from build123d import *

# Parameters (mm, degrees)
CYLINDER017_R          = 2.5
CYLINDER017_DEPTH      = 30
CYLINDER018_R          = 2.5
CYLINDER018_DEPTH      = 30
CYLINDER019_R          = 2.5
CYLINDER019_DEPTH      = 30
CYLINDER016_R          = 7.75
CYLINDER016_DEPTH      = 30
CYLINDER015_R          = 7.75
CYLINDER015_DEPTH      = 60
BOX001_W               = 20
BOX001_H               = 40
BOX001_DEPTH           = 20
CUT001_ROLL_ANGLE      = 180
CUT001_PLACEMENT_ANGLE = 90


with BuildPart() as taladros003:
    # Cylinder017 → Cylinder017 (new body)
    with BuildSketch(Plane(origin=(20, 15, 0), x_dir=(1, 0, 0), z_dir=(0, -1, 0))):
        Circle(CYLINDER017_R)
    extrude(amount=CYLINDER017_DEPTH)


with BuildPart() as taladros004:
    # Cylinder018 → Cylinder018 (new body)
    with BuildSketch(Plane(origin=(-20, 15, 0), x_dir=(1, 0, 0), z_dir=(0, -1, 0))):
        Circle(CYLINDER018_R)
    extrude(amount=CYLINDER018_DEPTH)


with BuildPart() as obj1:
    # Cylinder019 → Cylinder019 (new body)
    with BuildSketch(Plane(origin=(0, 15, 20), x_dir=(1, 0, 0), z_dir=(0, -1, 0))):
        Circle(CYLINDER019_R)
    extrude(amount=CYLINDER019_DEPTH)

    # Fusion004: union Taladros003, Taladros004
    add(taladros003.part)
    add(taladros004.part)


with BuildPart() as obj2:
    # Cylinder016 → Cylinder016 (new body)
    with BuildSketch(Plane.XY):
        Circle(CYLINDER016_R)
    extrude(amount=CYLINDER016_DEPTH)


with BuildPart() as obj3:
    # Cylinder015 → Cylinder015 (new body)
    with BuildSketch(Plane(origin=(-30, 0, 0), x_dir=(0, 0, -1), z_dir=(1, 0, 0))):
        Circle(CYLINDER015_R)
    extrude(amount=CYLINDER015_DEPTH)


with BuildPart() as obj4:
    # Box001 → Box001 (new body)
    with BuildSketch(Plane(origin=(-10, -30, -10), x_dir=(1, 0, 0), z_dir=(0, 0, 1))):
        with Locations((10, 20)):
            Rectangle(BOX001_W, BOX001_H)
    extrude(amount=BOX001_DEPTH)

    # Fusion003: union obj2, obj3
    add(obj2.part)
    add(obj3.part)

    # Cut001: cut obj1
    add(obj1.part, mode=Mode.SUBTRACT)


with BuildPart() as obj4_1:
    # Cut001 roll: moved
    add(obj4.part.rotate(Axis((0, 0, 0), (1, 0, 0)), CUT001_ROLL_ANGLE))


with BuildPart() as obj4_2:
    # Cut001 placement: moved
    add(obj4_1.part.moved(Location((11, -12, -22))).rotate(Axis((11, -12, -22), (0, 0, 1)), CUT001_PLACEMENT_ANGLE))


solid = obj4_2.part
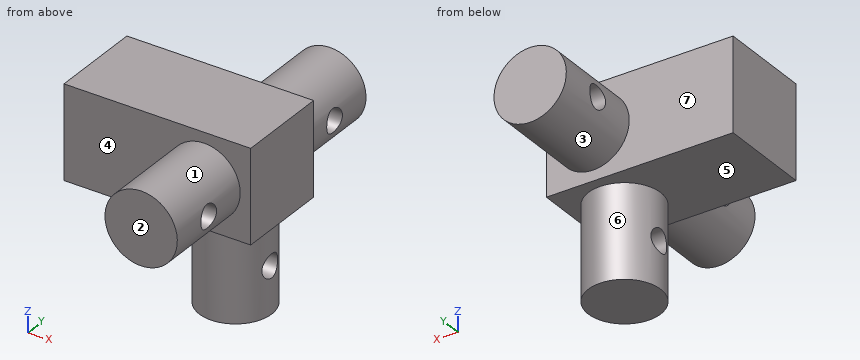
Source: CAD feature listing. Evaluate the final solid. Frame: model axes, mm. Face numbers are marked on the shaded views. A direction names the side the tool comes from. Round coordinates to 2 decimals unless told otherwise and drop trailing zeros. Order: outer loops, then holes, each group sorted by start corner. A loop starts at its lowest first (then second) coordinate and runs counter-clockwise, first axis right, second up. Notation, with made-up numbers: (-24, 11.25) - (30, 11.25) arc R19 cw to (30, 20.25) - close; hole circle Ø2 at (-0.5, -26.5). An arc over 180 degrees is marked (long way). Use a Markdown table: item, result. Add a question column.
1. Mould query, pull axis Y, two halves, no side actions, for the marked faces 4, 5, 6 and 7. Classes: +Y half, -Y half, draft (parallel to the pull), parting line (faces both ways), or undercut.
2. Section query A-A (z = -22). Return the cut outline in (x, y).
3. Section query C-C (x = 11). Return the cut outline in (y, z).
4. Section query D-D (y = -5.5). Return the cut outline in (x, z), then the cut area to 3 significant figures.
5. Set-up query: the marked faces 1, 2 and 3. Return all of +Z, -Z, +X, -X, +Y, -Y with unobstructed straight access to the full face (end or side cutting, diameter ignored); none if empty.
6. First-contact query: pin 1 (6 mm diameter, centred on y = -32, z = -22, fed in from +X); pin 2 (1.5 mm diameter, centred on x = 15, z = -36.5, fed in from +Y); pin 3 (6 mm diameter, centred on x = 0.5, z = -18.5, fed in from -Y). Flat tips, straight axial feed; report the tip coordinate or a pass-through.
7. Line query: probe 1 along Y at (x, z) = (7, -22); probe 2 along Z at (x, y) = (8.75, -12); probe 3 along Y at (x, z) = (10.5, -42). Output: solid intervals per line, ascending.
8. Section query B-B (y = -12). Return the cut outline in (x, z).
Derived:
| question | item | result |
|---|---|---|
| 1 | face 4 | -Y half |
| 1 | face 5 | draft |
| 1 | face 6 | parting line |
| 1 | face 7 | +Y half |
| 2 | outline | (-19, -22) - (3.25, -22) - (3.25, -29.5) - (18.75, -29.5) - (18.75, -22) - (21, -22) - (21, -2) - (18.75, -2) - (18.75, 5.5) - (3.25, 5.5) - (3.25, -2) - (-19, -2) - close; (3.25, -42) - (18.75, -42) - (18.75, -34.5) - (3.25, -34.5) - close; (3.25, 10.5) - (18.75, 10.5) - (18.75, 18) - (3.25, 18) - close |
| 3 | outline | (-42, -29.75) - (-22, -29.75) - (-22, -32) - (-19.75, -32) - (-19.75, -52) - (-4.25, -52) - (-4.25, -32) - (-2, -32) - (-2, -29.75) - (18, -29.75) - (18, -14.25) - (-2, -14.25) - (-2, -12) - (-22, -12) - (-22, -14.25) - (-42, -14.25) - close; hole circle Ø5 at (-32, -22); hole circle Ø5 at (-12, -42); hole circle Ø5 at (8, -22) |
| 4 | outline | (-19, -32) - (6.78, -32) - (6.78, -52) - (15.22, -52) - (15.22, -32) - (21, -32) - (21, -12) - (-19, -12) - close |
| 4 | area | 969 mm2 |
| 5 | face 1 | -Y |
| 5 | face 2 | +Z, -Z, +X, -X, -Y |
| 5 | face 3 | +Y |
| 6 | pin 1 | x = 18.75 |
| 6 | pin 2 | y = -4.96 |
| 6 | pin 3 | y = -22 |
| 7 | probe 1 | -42 to -34.5, -29.5 to 5.5, 10.5 to 18 |
| 7 | probe 2 | -52 to -44.5, -39.5 to -12 |
| 7 | probe 3 | -19.73 to -14.5, -9.5 to -4.27 |
| 8 | outline | (-19, -32) - (3.25, -32) - (3.25, -39.5) - (18.75, -39.5) - (18.75, -32) - (21, -32) - (21, -12) - (-19, -12) - close; (3.25, -52) - (18.75, -52) - (18.75, -44.5) - (3.25, -44.5) - close |
